```python
from build123d import *

# Parameters (mm, degrees)
F0_R     = 12.7
F0_R_2   = 44.45
F1_DEPTH = 25.4
F2_DEPTH = 25.4
F3_DEPTH = 25.4


with BuildPart() as f1:
    # F0 (on Front) → F1 (new body)
    with BuildSketch(Plane.XZ):
        with BuildLine():
            ThreePointArc((-69.75078125, -31.0881018641), (-59.174450896, -31.9106139737), (-50.6778846154, -38.2622792174))
            ThreePointArc((-50.6778846154, -38.2622792174), (0, -63.5), (50.6778846154, -38.2622792174))
            ThreePointArc((50.6778846154, -38.2622792174), (59.174450896, -31.9106139737), (69.75078125, -31.0881018641))
            ThreePointArc((69.75078125, -31.0881018641), (107.95, 0), (69.75078125, 31.0881018641))
            ThreePointArc((69.75078125, 31.0881018641), (59.174450896, 31.9106139737), (50.6778846154, 38.2622792174))
            ThreePointArc((50.6778846154, 38.2622792174), (0, 63.5), (-50.6778846154, 38.2622792174))
            ThreePointArc((-50.6778846154, 38.2622792174), (-59.174450896, 31.9106139737), (-69.75078125, 31.0881018641))
            ThreePointArc((-69.75078125, 31.0881018641), (-107.95, 0), (-69.75078125, -31.0881018641))
        make_face()
        with Locations((-76.2, 0)):
            Circle(F0_R, mode=Mode.SUBTRACT)
        Circle(F0_R_2, mode=Mode.SUBTRACT)
        with BuildLine():
            ThreePointArc((63.5, 0), (76.2, 12.7), (88.9, 0))
            ThreePointArc((88.9, 0), (76.2, -12.7), (63.5, 0))
        make_face(mode=Mode.SUBTRACT)
    extrude(amount=F1_DEPTH)

    # F0 (on Front) → F2 (join)
    with BuildSketch(Plane.XZ):
        with BuildLine():
            ThreePointArc((-69.75078125, -31.0881018641), (-59.174450896, -31.9106139737), (-50.6778846154, -38.2622792174))
            ThreePointArc((-50.6778846154, -38.2622792174), (0, -63.5), (50.6778846154, -38.2622792174))
            ThreePointArc((50.6778846154, -38.2622792174), (59.174450896, -31.9106139737), (69.75078125, -31.0881018641))
            ThreePointArc((69.75078125, -31.0881018641), (107.95, 0), (69.75078125, 31.0881018641))
            ThreePointArc((69.75078125, 31.0881018641), (59.174450896, 31.9106139737), (50.6778846154, 38.2622792174))
            ThreePointArc((50.6778846154, 38.2622792174), (0, 63.5), (-50.6778846154, 38.2622792174))
            ThreePointArc((-50.6778846154, 38.2622792174), (-59.174450896, 31.9106139737), (-69.75078125, 31.0881018641))
            ThreePointArc((-69.75078125, 31.0881018641), (-107.95, 0), (-69.75078125, -31.0881018641))
        make_face()
        with Locations((-76.2, 0)):
            Circle(F0_R, mode=Mode.SUBTRACT)
        Circle(F0_R_2, mode=Mode.SUBTRACT)
        with BuildLine():
            ThreePointArc((63.5, 0), (76.2, 12.7), (88.9, 0))
            ThreePointArc((88.9, 0), (76.2, -12.7), (63.5, 0))
        make_face(mode=Mode.SUBTRACT)
    extrude(amount=F2_DEPTH)

    # F0 (on Front) → F3 (cut)
    with BuildSketch(Plane.XZ):
        Circle(F0_R_2)
    extrude(amount=-F3_DEPTH, mode=Mode.SUBTRACT)


solid = f1.part
```
Geometry: final body of the model. Coordinates: model frame, mm. Round coordinates to 2 decimals unless told otherwise and drop trailing zeros. Order: outer loops, then holes, each group sorted by start corner. A loop starts at its lowest first (then second) coordinate and runs counter-clockwise, first axis right, second up. Notation, with made-up numbers: (-2, -23) -> (17, -23) arc R16 ccw to (17, 5) -> close; hole circle Ø7 at (72, 82.5). An arc over 180 degrees is marked (long way). Write each question's results on one line, items separated by ' | '.
Q1. Ray query, line 1 along Z through (x, y) = (76.2, -12.25); line 2 along Z through (x, y) = (-2, -3.75); line 3 along X through (y, z) = (-23.5, 9.5). Return the intervals inside material, ascending.
Response values:
line 1: -31.75 to -12.7, 12.7 to 31.75 | line 2: -63.47 to -44.4, 44.4 to 63.47 | line 3: -106.5 to -84.63, -67.77 to -43.42, 43.42 to 67.77, 84.63 to 106.5
Q2. Pin query (flat end, axial travel): pin 1 Ø10 at (y, z) = (-16.5, -25) entering from +X; pin 2 Ø8 at (x, y) = (20.5, -22.5) entering from +Z; pin 3 Ø3 at (x, y) = (86, -20.5) entering from -Z. Return the tip coordinate at first contact, or that it passes through.
Response values:
pin 1: x = 100.86 | pin 2: z = 61.32 | pin 3: z = -30.65
Q3. Section query A-A (z = 0). Output: boundary loops of the cut face in (x, y).
Response values:
outline: (-107.95, -25.4) -> (-88.9, -25.4) -> (-88.9, 0) -> (-107.95, 0) -> close; (-63.5, -25.4) -> (-44.45, -25.4) -> (-44.45, 0) -> (-63.5, 0) -> close; (44.45, -25.4) -> (63.5, -25.4) -> (63.5, 0) -> (44.45, 0) -> close; (88.9, -25.4) -> (107.95, -25.4) -> (107.95, 0) -> (88.9, 0) -> close
Q4. Section query B-B (x = -12.5). Output: boundary loops of the cut face in (y, z), and give its area (3 significant figures).
Response values:
outline: (-25.4, -62.26) -> (0, -62.26) -> (0, -42.66) -> (-25.4, -42.66) -> close; (-25.4, 42.66) -> (0, 42.66) -> (0, 62.26) -> (-25.4, 62.26) -> close | area: 996 mm²
Q5. Section query D-D (z = 20). Output: boundary loops of the cut face in (x, y).
Response values:
outline: (-100.86, -25.4) -> (-39.7, -25.4) -> (-39.7, 0) -> (-100.86, 0) -> close; (39.7, -25.4) -> (100.86, -25.4) -> (100.86, 0) -> (39.7, 0) -> close
Q6. Section query C-C (y = -5). Output: boundary loops of the cut face in (x, z), and give its area (3 significant figures).
Response values:
outline: (-69.75, -31.09) arc R19.05 cw to (-50.68, -38.26) arc R63.5 ccw to (50.68, -38.26) arc R19.05 cw to (69.75, -31.09) arc R31.75 ccw (long way) to (69.75, 31.09) arc R19.05 cw to (50.68, 38.26) arc R63.5 ccw to (-50.68, 38.26) arc R19.05 cw to (-69.75, 31.09) arc R31.75 ccw (long way) to start; hole circle Ø25.4 at (-76.2, 0); hole circle Ø88.9 at (0, 0); hole circle Ø25.4 at (76.2, 0) | area: 10,600 mm²
Q7. Pull-direction query (X, two-part tool) for faces 1 (the face through (46, 0, 1)), 2 (the face through (-59.316, -12.522, -31.858)), 3 (the face through (-59.034, -12.522, 31.964)), 4 (the face through (-0.821, -12.522, -63.495)); classes: released by +X, released by -X, zero draft, split by the parting line, or undercut.
Response values:
face 1: zero draft | face 2: undercut | face 3: undercut | face 4: split by the parting line
